Part model, mm, in its own coordinate system. A direction names the side the tool comes from. Give positions to 0.01 mm unless a question says otherwise; leave off trailing zeros. Order: outer loops, then holes, each group sorted by start corner. A loop starts at its lowest first (then second) coordinate and runs counter-clockwise, first axis right, second up. Notation, with made-up numbers: (-1.75, 67) - (45.25, 67) arc R24 cw to (45.25, 98) - close; hole circle Ø10 at (-12, 5.5). An arc over 180 degrees is marked (long way). Use a Markdown table: item, result. Add a question column.
from build123d import *
from OCP.BRepFilletAPI import BRepFilletAPI_MakeChamfer

# Parameters (mm, degrees)
P_IDAT_VYSUNUT_M5_DEPTH = 1.6
P_IDAT_VYSUNUT_M6_DEPTH = 2
SKICA2_7_W              = 2
SKICA2_7_H              = 2
P_IDAT_VYSUNUT_M7_DEPTH = 1
P_IDAT_VYSUNUT_M8_DEPTH = 1
ZKOSEN_5_SIZE2          = 1.678199262
ZKOSEN_5_SIZE           = 2
ZKOSEN_8_SIZE2          = 2
ZKOSEN_8_SIZE           = 1.678199262
ZKOSEN_12_SIZE          = 1.461883237
ZKOSEN_12_SIZE_2        = 1
ZKOSEN_12_SIZE_3        = 0.577350269


with BuildPart() as part:
    # Skica1 → Přidat vysunutím5 (new body)
    with BuildSketch(Plane.XY):
        Polygon((0, 0), (0, 20), (-12.412784718, 31.615626352), (-23, 25), (-23, 0), align=None)
    extrude(amount=P_IDAT_VYSUNUT_M5_DEPTH)

    # Skica2 → Přidat vysunutím6 (add)
    with BuildSketch(Plane.XY.offset(1.6)):
        Polygon((-17, 25.95626352), (-17, 12), (-15, 12), (-11.502481599, 12), align=None)
        Polygon((-22.497518401, 12), (-19, 12), (-17, 12), (-17, 25.95626352), align=None)
    extrude(amount=P_IDAT_VYSUNUT_M6_DEPTH)

    # Skica2<7> → Přidat vysunutím7 (add)
    with BuildSketch(Plane.XY.offset(1.6)):
        with Locations((-16, 11)):
            Rectangle(SKICA2_7_W, SKICA2_7_H)
        with Locations((-18, 11)):
            Rectangle(SKICA2_7_W, SKICA2_7_H)
    extrude(amount=P_IDAT_VYSUNUT_M7_DEPTH)

    # Skica3 → Přidat vysunutím8 (add)
    with BuildSketch(Plane.XY.offset(1.6)):
        with BuildLine():
            Line((-3.705128205, 4.115384615), (-3.705128205, 2))
            Line((-3.705128205, 2), (-10.897435897, 2))
            add(Edge.make_bspline(
                [(-10.897435897, 2), (-10.87308441, 2.180790308), (-10.824395089, 2.542269551), (-10.673865117, 3.070299742), (-10.472959166, 3.585566992), (-10.254913916, 4.004869463), (-10.038043764, 4.342393523), (-9.841277463, 4.618963346), (-9.60654249, 4.913221767), (-9.337245105, 5.227544267), (-9.034873554, 5.562913411), (-8.697171951, 5.918082368), (-8.322529407, 6.291350846), (-8.058961705, 6.54481851), (-7.922676282, 6.67588141)],
                knots=[0, 0, 0, 0, 1.156289446, 2.311930546, 3.473459201, 4.661751613, 5.303057008, 6.018253237, 6.81459331, 7.690699809, 8.644447906, 9.679642995, 10.800191253, 12, 12, 12, 12], degree=3))
            add(Edge.make_bspline(
                [(-7.922676282, 6.67588141), (-7.813918956, 6.780862005), (-7.606877039, 6.980714138), (-7.312048947, 7.266894293), (-7.052864674, 7.529975199), (-6.823905036, 7.763139303), (-6.630459323, 7.972323552), (-6.469982936, 8.154242742), (-6.34044346, 8.309637702), (-6.270284768, 8.408220362), (-6.239182692, 8.451923077)],
                knots=[0, 0, 0, 0, 1.480720495, 2.818855715, 4.024636094, 5.098235712, 6.019786162, 6.815086302, 7.474715479, 8, 8, 8, 8], degree=3))
            add(Edge.make_bspline(
                [(-6.239182692, 8.451923077), (-6.175493233, 8.557718073), (-6.052643645, 8.761784362), (-5.91792888, 9.082682292), (-5.837068057, 9.403513936), (-5.825971765, 9.617891805), (-5.820512821, 9.723357372)],
                knots=[0, 0, 0, 0, 1.0911822, 2.104764037, 3.067617678, 4, 4, 4, 4], degree=3))
            add(Edge.make_bspline(
                [(-5.820512821, 9.723357372), (-5.824474653, 9.833108474), (-5.831970132, 10.040748999), (-5.894821019, 10.333768175), (-6.006276867, 10.585659667), (-6.15973106, 10.797196661), (-6.353774193, 10.962935085), (-6.580616259, 11.085399693), (-6.843577862, 11.153106661), (-7.028402789, 11.16201224), (-7.125, 11.166666667)],
                knots=[0, 0, 0, 0, 1.193122327, 2.257294386, 3.237245624, 4.168877528, 5.075331632, 5.990371598, 6.949684428, 8, 8, 8, 8], degree=3))
            add(Edge.make_bspline(
                [(-7.125, 11.166666667), (-7.220944609, 11.16231978), (-7.406288878, 11.153922533), (-7.669703299, 11.080565334), (-7.900142302, 10.953576306), (-8.06436539, 10.808860058), (-8.175305876, 10.668134018), (-8.250896853, 10.545500545), (-8.316050374, 10.406151312), (-8.37378183, 10.251655158), (-8.419383153, 10.080242168), (-8.456107626, 9.893217825), (-8.485702239, 9.689575671), (-8.495113848, 9.547907653), (-8.5, 9.474358974)],
                knots=[0, 0, 0, 0, 1.402788338, 2.709884207, 3.961032948, 5.225417836, 5.883680772, 6.578928686, 7.329201998, 8.132101139, 8.990263233, 9.922304639, 10.921339128, 12, 12, 12, 12], degree=3))
            Line((-8.5, 9.474358974), (-10.615384615, 9.681490385))
            add(Edge.make_bspline(
                [(-10.615384615, 9.681490385), (-10.598377251, 9.824305509), (-10.565402688, 10.101201217), (-10.483114114, 10.498918926), (-10.378898684, 10.865831465), (-10.247788098, 11.201257911), (-10.095201314, 11.507331251), (-9.913355139, 11.779458664), (-9.708603468, 12.020654551), (-9.480769352, 12.230790543), (-9.231301205, 12.410535137), (-8.969529148, 12.57098477), (-8.690337423, 12.702604473), (-8.396799939, 12.811078884), (-8.089049352, 12.897770766), (-7.765662274, 12.955090263), (-7.42863453, 12.995409017), (-7.198577984, 12.998446608), (-7.080929487, 13)],
                knots=[0, 0, 0, 0, 1.270971563, 2.464210789, 3.586263665, 4.638946707, 5.643716971, 6.603612468, 7.52484387, 8.434700188, 9.336036235, 10.239171475, 11.145359471, 12.059630629, 13.003312604, 13.96741569, 14.960557767, 16, 16, 16, 16], degree=3))
            add(Edge.make_bspline(
                [(-7.080929487, 13), (-6.953030371, 12.997541845), (-6.703930784, 12.992754281), (-6.34028961, 12.953218534), (-5.998674853, 12.884282231), (-5.676099879, 12.79296634), (-5.375877361, 12.67105295), (-5.095505554, 12.52366473), (-4.83939702, 12.345207999), (-4.603734114, 12.145414763), (-4.393070332, 11.925706984), (-4.20854792, 11.691351493), (-4.053955652, 11.442511564), (-3.924228998, 11.182220281), (-3.827907833, 10.90628918), (-3.757724044, 10.618533633), (-3.711189366, 10.317611197), (-3.707170936, 10.112088), (-3.705128205, 10.007612179)],
                knots=[0, 0, 0, 0, 1.210756838, 2.35810096, 3.457354827, 4.507168606, 5.527358126, 6.519769748, 7.499700793, 8.476517721, 9.440526811, 10.376769937, 11.295256217, 12.209626307, 13.124630862, 14.055668209, 15.011616881, 16, 16, 16, 16], degree=3))
            add(Edge.make_bspline(
                [(-3.705128205, 10.007612179), (-3.707819477, 9.887707131), (-3.713158546, 9.649833916), (-3.764276175, 9.298186238), (-3.84237396, 8.954647512), (-3.957796338, 8.618378159), (-4.104103161, 8.28131186), (-4.292696164, 7.942692037), (-4.511666905, 7.592306518), (-4.683112364, 7.36576699), (-4.771634615, 7.248798077)],
                knots=[0, 0, 0, 0, 0.953409949, 1.89141903, 2.821310783, 3.752688675, 4.715703262, 5.740811754, 6.833515735, 8, 8, 8, 8], degree=3))
            add(Edge.make_bspline(
                [(-4.771634615, 7.248798077), (-4.80509214, 7.206658226), (-4.876750403, 7.116404431), (-4.998659939, 6.978014195), (-5.139942605, 6.826848432), (-5.298602846, 6.660077667), (-5.479881522, 6.483607708), (-5.677256214, 6.290058721), (-5.899411985, 6.089331377), (-6.12951153, 5.876418507), (-6.360611244, 5.669193404), (-6.5730252, 5.472375498), (-6.765967752, 5.298233923), (-6.930453202, 5.137155265), (-7.076156545, 5.000133027), (-7.197826149, 4.880140867), (-7.29773874, 4.780083699), (-7.43541186, 4.624119958), (-7.610585282, 4.413178934), (-7.733826947, 4.21161882), (-7.792668269, 4.115384615)],
                knots=[0, 0, 0, 0, 0.665555651, 1.425465941, 2.280616993, 3.225313414, 4.272635571, 5.410053715, 6.644756443, 7.976022804, 9.288331007, 10.484517221, 11.558462543, 12.503158964, 13.33222979, 14.032602617, 14.617328242, 15.080653724, 16.606167857, 18, 18, 18, 18], degree=3))
            Line((-7.792668269, 4.115384615), (-3.705128205, 4.115384615))
        make_face()
    extrude(amount=P_IDAT_VYSUNUT_M8_DEPTH)

    # Zkosení5
    zkosen_5_edges = [part.edges().sort_by_distance(p)[0] for p in [
        (-14.2512408, 18.97813176, 3.6),
    ]]
    zkosen_5_side = [part.faces().sort_by_distance(p)[0] for p in [
        (-14.2512408, 18.97813176, 3.566436015),
    ]]
    chamfer(zkosen_5_edges, length=ZKOSEN_5_SIZE - 0.0001, length2=ZKOSEN_5_SIZE2 - 0.0001, reference=zkosen_5_side[0])  # a hair under: the kernel refuses the full size

    # Zkosení8
    zkosen_8_edges = [part.edges().sort_by_distance(p)[0] for p in [
        (-20.1996587, 17.833456695, 3.6),
    ]]
    zkosen_8_side = [part.faces().sort_by_distance(p)[0] for p in [
        (-20.168430178, 17.821155453, 3.6),
    ]]
    chamfer(zkosen_8_edges, length=ZKOSEN_8_SIZE - 0.0001, length2=ZKOSEN_8_SIZE2 - 0.0001, reference=zkosen_8_side[0])  # a hair under: the kernel refuses the full size

    # Zkosení12
    zkosen_12_edges_1 = [part.edges().sort_by_distance(p)[0] for p in [
        (-15.153039798, 16.68878163, 3.6),
    ]]
    zkosen_12_side_1 = [part.faces().sort_by_distance(p)[0] for p in [
        (-15.171648149, 16.681451605, 3.6),
    ]]
    zkosen_12_edges_2 = [part.edges().sort_by_distance(p)[0] for p in [
        (-17, 12, 3.6),
    ]]
    zkosen_12_side_2 = [part.faces().sort_by_distance(p)[0] for p in [
        (-17, 12, 3.588452995),
    ]]
    zkosen_12_edges_3 = [part.edges().sort_by_distance(p)[0] for p in [
        (-18.846960202, 16.68878163, 3.6),
    ]]
    zkosen_12_side_3 = [part.faces().sort_by_distance(p)[0] for p in [
        (-18.828351851, 16.681451605, 3.6),
    ]]
    zkosen_12 = BRepFilletAPI_MakeChamfer(part.part.solid().wrapped)
    for e in zkosen_12_edges_1:
        zkosen_12.Add(ZKOSEN_12_SIZE - 0.0001, ZKOSEN_12_SIZE_2 - 0.0001, e.wrapped, zkosen_12_side_1[0].wrapped)
    for e in zkosen_12_edges_2:
        zkosen_12.Add(ZKOSEN_12_SIZE_2 - 0.0001, ZKOSEN_12_SIZE_3 - 0.0001, e.wrapped, zkosen_12_side_2[0].wrapped)
    for e in zkosen_12_edges_3:
        zkosen_12.Add(ZKOSEN_12_SIZE - 0.0001, ZKOSEN_12_SIZE_2 - 0.0001, e.wrapped, zkosen_12_side_3[0].wrapped)
    add(Compound.cast(zkosen_12.Shape()), mode=Mode.REPLACE)  # a hair under: the kernel refuses the full size


solid = part.part
1. Cut at C-C (z = 0.65). Write the cut outline in (x, y), plus the area to 3 significant figures.
2. Mould opens along X. For faces 1 (the face through (-17.06, 12.23, 3)), 2 (the face through (-19.235, 18.889, 2.208)), 3 (the face through (-15, 11, 2)) say: released by +X, released by -X, zero draft, split by the parting line, or undercut.
3. Drill centre lines: probe 1 along Z at (x, y) = (-3.5, 4); probe 2 along Y at (x, z) = (-4.75, 1.3); probe 3 along Y at (x, z) = (-8.5, 1.3). Where is each one in solid material? Low to high. Write a range as [from, to].
4. Tool access for faces 4 (the face through (-14.6, 12, 2.1)), 5 (the face through (-6, 4.115, 2)), 6 (the face through (-17, 11, 2.6)): list every direction of +Z, -Z, +X, -X, +Y, -Y with a clear straight run to the whole face (end or side of a thin tool).
5. Pin check, flat tips, straight feed: P1, Ø10, axis at x = -2.5, y = 12, coming from the +Z side; P2, Ø0.8, axis at y = 10.5, z = 2.5, coming from the +X side; P3, Ø0.5, axis at x = -17.5, z = 2, coming from the -Y side. Stop position of each tip, or through.
Responses:
| question | item | result |
|---|---|---|
| 1 | outline | (-23, 0) - (0, 0) - (0, 20) - (-12.41, 31.62) - (-23, 25) - close |
| 1 | area | 620 mm² |
| 2 | face 1 | zero draft |
| 2 | face 2 | released by -X |
| 2 | face 3 | undercut |
| 3 | probe 1 | z = [0, 1.6] |
| 3 | probe 2 | y = [0, 24.44] |
| 3 | probe 3 | y = [0, 27.95] |
| 4 | face 4 | +Z, -Y |
| 4 | face 5 | +Z, +X |
| 4 | face 6 | +Z, +X, -X, -Y |
| 5 | P1 | stops at z = 2.6 |
| 5 | P2 | stops at x = -3.71 |
| 5 | P3 | stops at y = 10 |
